```python
from build123d import *

# Parameters (mm, degrees)
AUFSATZ_LINEAR_START                        = -8.5
AUFSATZ_LINEAR_AUSTRAGEN1_DEPTH             = 41
VERRUNDUNG1_R                               = 0.5
FORMSENKUNG_F_R_M5_SENKSCHRAUBE_MIT_2_COUNT = 2
FORMSENKUNG_F_R_M5_SENKSCHRAUBE_MIT_2_PITCH = 173


with BuildPart() as part:
    # Skizze1 → Aufsatz-Linear austragen1 (new body)
    with BuildSketch(Plane.XY.offset(AUFSATZ_LINEAR_START)):
        with BuildLine():
            Line((225, 23), (426.559028492, 23))
            ThreePointArc((426.559028492, 23), (422.879511457, 21.29187069), (419.532291702, 19))
            Line((419.532291702, 19), (417.992648648, 19))
            Line((417.992648648, 19), (225, 19))
            Line((225, 19), (225, 23))
        make_face()
    extrude(amount=-AUFSATZ_LINEAR_AUSTRAGEN1_DEPTH)

    # Verrundung1
    verrundung1_edges = [part.edges().sort_by_distance(p)[0] for p in [
        (225, 23, -29),
        (426.559028492, 23, -29),
        (419.532291702, 19, -29),
        (225, 19, -29),
    ]]
    fillet(verrundung1_edges, radius=VERRUNDUNG1_R)

    # Skizze5 → Formsenkung für M5 Senkschraube mit Innensechskant1 (revolve, cut)
    with BuildSketch(Plane(origin=(398, 23, -19.5), x_dir=(0, 0, 1), z_dir=(1, 0, 0))):
        Polygon((0, 0), (0, 5.652366702), (2.75, 4), (2.75, 4.485), (5.735, 1.5), (5.735, 0), align=None)
    formsenkung_f_r_m5_senkschraube_mit_inne = revolve(axis=Axis((398, 29.35, -19.5), (0, -1, 0)), mode=Mode.SUBTRACT)

    # Formsenkung f_r M5 Senkschraube mit  2: Formsenkung für M5 Senkschraube mit Innensechskant1 ×2
    with Locations(*[(-i * FORMSENKUNG_F_R_M5_SENKSCHRAUBE_MIT_2_PITCH, 0, 0) for i in range(1, FORMSENKUNG_F_R_M5_SENKSCHRAUBE_MIT_2_COUNT)]):
        add(formsenkung_f_r_m5_senkschraube_mit_inne, mode=Mode.SUBTRACT)

    # Spiegeln1: part across plane


with BuildPart() as part_1:
    add(part.part)
    add(part.part.mirror(Plane(origin=(435, 0, -49.5), x_dir=(1, 0, 0), z_dir=(0, 0, 1))))


solid = part_1.part
```
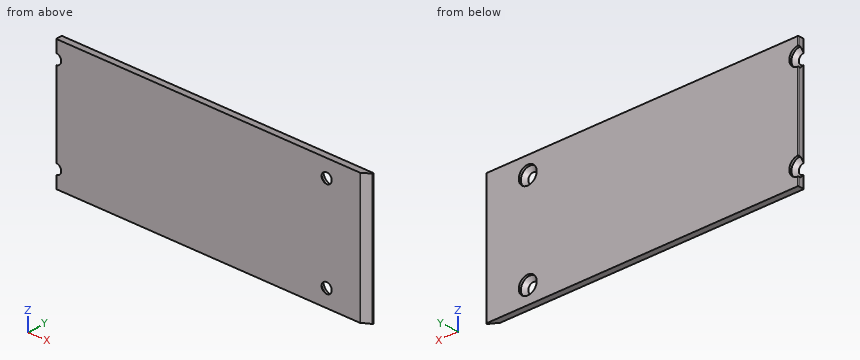
Check sheet for the modelled part. Datum: model origin and axes. Units: mm. Give positions to 0.01 mm unless a question says otherwise; leave off trailing zeros. Order: outer loops, then holes, each group sorted by start corner. A loop starts at its lowest first (then second) coordinate and runs counter-clockwise, first axis right, second up. Notation, with made-up numbers: M 68.5,-37.75 L 98.5,-37.75 A13 ccw 98.5,-23.75 Z; hole C 56,17 d8. An arc over 180 degrees is marked long. Answer in a Markdown table with one row per item.
1) Gauge pin test, flat ends, axial feed: P1, Ø9, axis at x = 398, z = -79.5, coming from the +Y side (3 decimals); P2, Ø13, axis at x = 398, z = -19.5, coming from the +Y side. Record the tip position at first contact, or that the pin passes through.
Filled sheet:
| item | result |
|---|---|
| P1 | stops at y = 20.265 |
| P2 | stops at y = 23 |
2) Cross-section at A-A, the plane x = 398. Enter the section's corners in (y, z) (3 decimals), plus the area to 3 significant figures.
Filled sheet:
| item | result |
|---|---|
| outline | M 19,-90.5 L 23,-90.5 L 23,-85.235 L 21.5,-85.235 L 19,-82.735 Z; M 19,-76.265 L 21.5,-73.765 L 23,-73.765 L 23,-25.235 L 21.5,-25.235 L 19,-22.735 Z; M 19,-16.265 L 21.5,-13.765 L 23,-13.765 L 23,-8.5 L 19,-8.5 Z |
| area | 249 mm2 |
3) Thickness scan on L1, parallel to Z at x = 398, y = 22 (3 decimals); L2, parallel to X at y = 21.95, z = -19.5 (3 decimals); L3, parallel to Z at x = 399.5, y = 22.6. Record the ranges inside material, lowest first. Write a range as [from, to].
Filled sheet:
| item | result |
|---|---|
| L1 | z = [-90.5, -85.235], [-73.765, -25.235], [-13.765, -8.5] |
| L2 | x = [230.735, 392.265], [403.735, 424.117] |
| L3 | z = [-90.5, -85.04], [-73.96, -25.04], [-13.96, -8.5] |
4) Cross-section at B-B, the plane z = -19.5. Enter the section's corners in (x, y) (3 decimals).
Filled sheet:
| item | result |
|---|---|
| outline | M 228.235,19 L 394.765,19 L 392.265,21.5 L 392.265,23 L 230.735,23 L 230.735,21.5 Z; M 401.235,19 L 419.356,19 A0.5 ccw 419.668,19.11 A24.5 cw 424.321,22.05 A0.5 ccw 424.103,23 L 403.735,23 L 403.735,21.5 Z |
